For this review, take the finished solid that the model builds, in its own axes (mm). A direction names the side the tool comes from. Round coordinates to 2 decimals unless told otherwise and drop trailing zeros. Loops run counter-clockwise (first coordinate to the right, second up) from the corner with the lowest first, then second, coordinate; pieces in that order, holes last.
Autodesk Inventor part; units mm, degrees
ref_plane "YZ Plane" through (0, 0, 0) normal (1, 0, 0) x (0, 1, 0)
ref_plane "XZ Plane" through (0, 0, 0) normal (0, 1, 0) x (-1, 0, 0)
ref_plane "XY Plane" through (0, 0, 0) normal (0, 0, 1) x (1, 0, 0)
sketch "Sketch1" plane through (0, 0, 0) normal (0, 1, 0) x (-1, 0, 0)
  line L0 (-500, 350) -> (500, 350)
  line L1 (500, 350) -> (500, -350)
  line L2 (500, -350) -> (-500, -350)
  line L3 (-500, -350) -> (-500, 350)
  line L4 (-500, 350) -> (500, -350) construction
  line L5 (500, 350) -> (-500, -350) construction
  line L6 (500, -350) -> (-50, -350)
  line L7 (-50, -350) -> (-50, 350)
  line L8 (-50, 350) -> (500, 350)
  line L9 (500, 350) -> (500, -350)
  line L10 (500, -350) -> (450, -350)
  line L11 (450, -350) -> (450, 350)
  line L12 (450, 350) -> (500, 350)
  line L13 (500, 350) -> (500, -350)
  line L14 (0, -350) -> (-50, -350)
  line L15 (-50, -350) -> (-50, 350)
  line L16 (-50, 350) -> (0, 350)
  line L17 (0, 350) -> (0, -350)
  point P0 (0, 0)
  point P1 (450, 350)
  dimension "d0" = 1000
  dimension "d1" = 700
  dimension "d2" = 550
  dimension "d3" = 50
  dimension "d4" = 50
extrude "Extrusion1" add sketch "Sketch1" along normal blind 110 contours L0 L17 L2 L7 | L0 L1 L2 L11
extrude "Extrusion2" add sketch "Sketch1" along normal blind 30 contours L0 L7 L2 L3 | L0 L11 L2 L17
sketch "Sketch2" plane through (0, 0, 0) normal (0, -1, 0) x (1, 0, 0)
  line L0 (500, -350) -> (50, -350)
  line L1 (500, -350) -> (450, -350)
  line L2 (450, -350) -> (450, -300)
  line L3 (450, -300) -> (500, -300)
  line L4 (500, -300) -> (500, -350)
  line L5 (50, 350) -> (500, 350)
  line L6 (500, 300) -> (450, 300)
  line L7 (450, 300) -> (450, 350)
  line L8 (450, 350) -> (500, 350)
  line L9 (500, 350) -> (500, 300)
  line L10 (-500, -350) -> (-500, 350)
  line L11 (-500, -350) -> (-450, -350)
  line L12 (-450, -350) -> (-450, -300)
  line L13 (-450, -300) -> (-500, -300)
  line L14 (-500, -300) -> (-500, -350)
  line L15 (-500, 350) -> (-450, 350)
  line L16 (-450, 350) -> (-450, 300)
  line L17 (-450, 300) -> (-500, 300)
  line L18 (-500, 300) -> (-500, 350)
  point P0 (0, 0)
  dimension "d9" = 50
  dimension "d10" = 50
  dimension "d11" = 50
  dimension "d12" = 50
  dimension "d13" = 50
  dimension "d14" = 50
  dimension "d15" = 50
  dimension "d16" = 50
extrude "Extrusion3" add sketch "Sketch2" along normal blind 500
sketch "Sketch3" plane through (0, 30, 0) normal (0, 1, 0) x (1, 0, 0)
  line L0 (-450, -350) -> (-450, 350)
  line L1 (-450, 350) -> (-300, 350)
  line L2 (-300, 350) -> (-300, -350)
  line L3 (-300, -350) -> (-150, -350)
  line L4 (-150, -350) -> (-150, 350)
  line L5 (-150, 350) -> (0, 350)
  line L6 (0, 350) -> (0, -350)
  line L7 (0, 350) -> (0, -350)
  line L8 (0, -350) -> (-450, -350)
  line L9 (-450, -350) -> (-450, 350)
  line L10 (-150, 350) -> (-300, 350)
  line L11 (-450, 175) -> (0, 175)
  line L12 (-450, 0) -> (0, 0)
  line L13 (0, 350) -> (-450, 350)
  line L14 (-450, -175) -> (0, -175)
  line L15 (-430, 330) -> (-320, 330)
  line L16 (-320, 330) -> (-320, 195)
  line L17 (-320, 195) -> (-430, 195)
  line L18 (-430, 195) -> (-430, 330)
  line L19 (-280, 330) -> (-170, 330)
  line L20 (-170, 330) -> (-170, 195)
  line L21 (-170, 195) -> (-280, 195)
  line L22 (-280, 195) -> (-280, 330)
  line L23 (-130, 330) -> (-20, 330)
  line L24 (-20, 330) -> (-20, 195)
  line L25 (-20, 195) -> (-130, 195)
  line L26 (-130, 195) -> (-130, 330)
  line L27 (-430, 155) -> (-320, 155)
  line L28 (-320, 155) -> (-320, 20)
  line L29 (-320, 20) -> (-430, 20)
  line L30 (-430, 20) -> (-430, 155)
  line L31 (-280, 155) -> (-170, 155)
  line L32 (-170, 155) -> (-170, 20)
  line L33 (-170, 20) -> (-280, 20)
  line L34 (-280, 20) -> (-280, 155)
  line L35 (-130, 155) -> (-20, 155)
  line L36 (-20, 155) -> (-20, 20)
  line L37 (-20, 20) -> (-130, 20)
  line L38 (-130, 20) -> (-130, 155)
  line L39 (-430, -20) -> (-320, -20)
  line L40 (-320, -20) -> (-320, -155)
  line L41 (-320, -155) -> (-430, -155)
  line L42 (-430, -155) -> (-430, -20)
  line L43 (-280, -20) -> (-170, -20)
  line L44 (-170, -20) -> (-170, -155)
  line L45 (-170, -155) -> (-280, -155)
  line L46 (-280, -155) -> (-280, -20)
  line L47 (-130, -20) -> (-20, -20)
  line L48 (-20, -20) -> (-20, -155)
  line L49 (-20, -155) -> (-130, -155)
  line L50 (-130, -155) -> (-130, -20)
  line L51 (-430, -195) -> (-320, -195)
  line L52 (-320, -195) -> (-320, -330)
  line L53 (-320, -330) -> (-430, -330)
  line L54 (-430, -330) -> (-430, -195)
  line L55 (-280, -195) -> (-170, -195)
  line L56 (-170, -195) -> (-170, -330)
  line L57 (-170, -330) -> (-280, -330)
  line L58 (-280, -330) -> (-280, -195)
  line L59 (-130, -195) -> (-20, -195)
  line L60 (-20, -195) -> (-20, -330)
  line L61 (-20, -330) -> (-130, -330)
  line L62 (-130, -330) -> (-130, -195)
  point P0 (0, 0)
  point P1 (-280, 87.5)
  point P2 (-225, 20)
  point P3 (-225, -195)
  dimension "d19" = 150
  dimension "d20" = 150
  dimension "d21" = 150
  dimension "d22" = 0
  dimension "d23" = 700
  dimension "d24" = 175
  dimension "d25" = 175
  dimension "d26" = 175
  dimension "d27" = 175
  dimension "d28" = 20
  dimension "d29" = 20
  dimension "d30" = 20
  dimension "d31" = 20
  dimension "d32" = 20
  dimension "d33" = 20
  dimension "d34" = 20
  dimension "d35" = 20
  dimension "d36" = 110
  dimension "d37" = 110
  dimension "d38" = 20
  dimension "d39" = 20
  dimension "d40" = 20
  dimension "d41" = 20
  dimension "d42" = 20
  dimension "d43" = 20
  dimension "d44" = 20
  dimension "d45" = 20
  dimension "d46" = 20
  dimension "d47" = 20
  dimension "d48" = 20
  dimension "d49" = 20
extrude "Extrusion4" add sketch "Sketch3" along normal blind 20
properties part number "Table_2"
(1) Add section B-B (y = 71.5). Give the boundary of the cut face in (x, z), plus the area to 3 significant figures.
(2) For L1, parallel to X at y = -378.5, z = -301.5; L2, parallel to Y at x = -434, z = 6.5; L3, parallel to Y at x = -189.5, z = 143, list the stretches that pass through material, from the lowest coordinate up.
(3) Add section A-A (y = -100.5). Give the boundary of the cut face in (x, z), plus the area to 3 significant figures.
(4) Add section D-D (x = -384). Give the boundary of the cut face in (y, z).
(5) Add section C-C (z = -288.5). Give the boundary of the cut face in (x, y).
(6) Insertion check: pin 1 Ø6 at (y, z) = (40, -78.5) entering from +X; pin 2 Ø12 at (x, z) = (154.5, 198.5) entering from +Y; pin 3 Ø12 at (x, z) = (-109, -254.5) entering from -Y. Each pin has a flat end and moves straight along its axis. Give the tip position at first contact, or say it passes through.
(7) The part is to be moulded in two halves that separate along X. For faces 1 (the flat face through (-475, 110, 5)), 2 (the flat face through (500, 19, -2)), 3 (the flat face through (450, -246, 325)), say which applies: pulls with the +X half, pulls with the -X half, needs draft (parallel to the pull), parting line crosses it, or undercut.
(8) For faces 4 (the flat face through (278, 30, 5)), 5 (the flat face through (0, 80, 5)), 6 (the flat face through (-224, 30, 263)), 7 (the flat face through (475, -246, -300)), list the 3-axis set-ups (+Z, -Z, +X, -X, +Y, -Y) from which the entire face can be reached by the end or side of a thin tool; tool diameter is ignored.
Outcome:
1. outline: (-500, -350) - (-450, -350) - (-450, 350) - (-500, 350) - close; (0, -350) - (50, -350) - (50, 350) - (0, 350) - close
1. area: 70,000 mm2
2. L1: x = -500 to -450, 450 to 500
2. L2: y = 0 to 50
2. L3: y = 0 to 30
3. outline: (-500, -350) - (-450, -350) - (-450, -300) - (-500, -300) - close; (-500, 300) - (-450, 300) - (-450, 350) - (-500, 350) - close; (450, -350) - (500, -350) - (500, -300) - (450, -300) - close; (450, 300) - (500, 300) - (500, 350) - (450, 350) - close
3. area: 10,000 mm2
4. outline: (0, -350) - (50, -350) - (50, -330) - (30, -330) - (30, -195) - (50, -195) - (50, -155) - (30, -155) - (30, -20) - (50, -20) - (50, 20) - (30, 20) - (30, 155) - (50, 155) - (50, 195) - (30, 195) - (30, 330) - (50, 330) - (50, 350) - (0, 350) - close
5. outline: (-500, 0) - (500, 0) - (500, 30) - (50, 30) - (50, 110) - (0, 110) - (0, 50) - (-20, 50) - (-20, 30) - (-130, 30) - (-130, 50) - (-170, 50) - (-170, 30) - (-280, 30) - (-280, 50) - (-320, 50) - (-320, 30) - (-430, 30) - (-430, 50) - (-450, 50) - (-450, 110) - (-500, 110) - close
6. pin 1: stops at x = 50
6. pin 2: stops at y = 30
6. pin 3: stops at y = 0
7. face 1: needs draft
7. face 2: pulls with the +X half
7. face 3: undercut
8. face 4: +Z, -Z, +X, +Y
8. face 5: +Z, -Z, +Y
8. face 6: +Y
8. face 7: +X, -X, -Y
